Verification items for this drawing (mm, ordinates from the low corner). Round coordinates to 2 decimals unless told otherwise and drop trailing zeros. Write each loop counter-clockwise with the first axis right and the second up, starting at its lowest first coordinate (ties: lowest second). Pieces come first, ordered by that corner, then holes. Notation, with made-up numbers: (64, 7.5) -> (113, 7.5) arc R18 cw to (113, 33.5) -> close; hole circle Ø5 at (63.25, 17.25). An arc over 180 degrees is marked (long way). One line per item, written item: value.
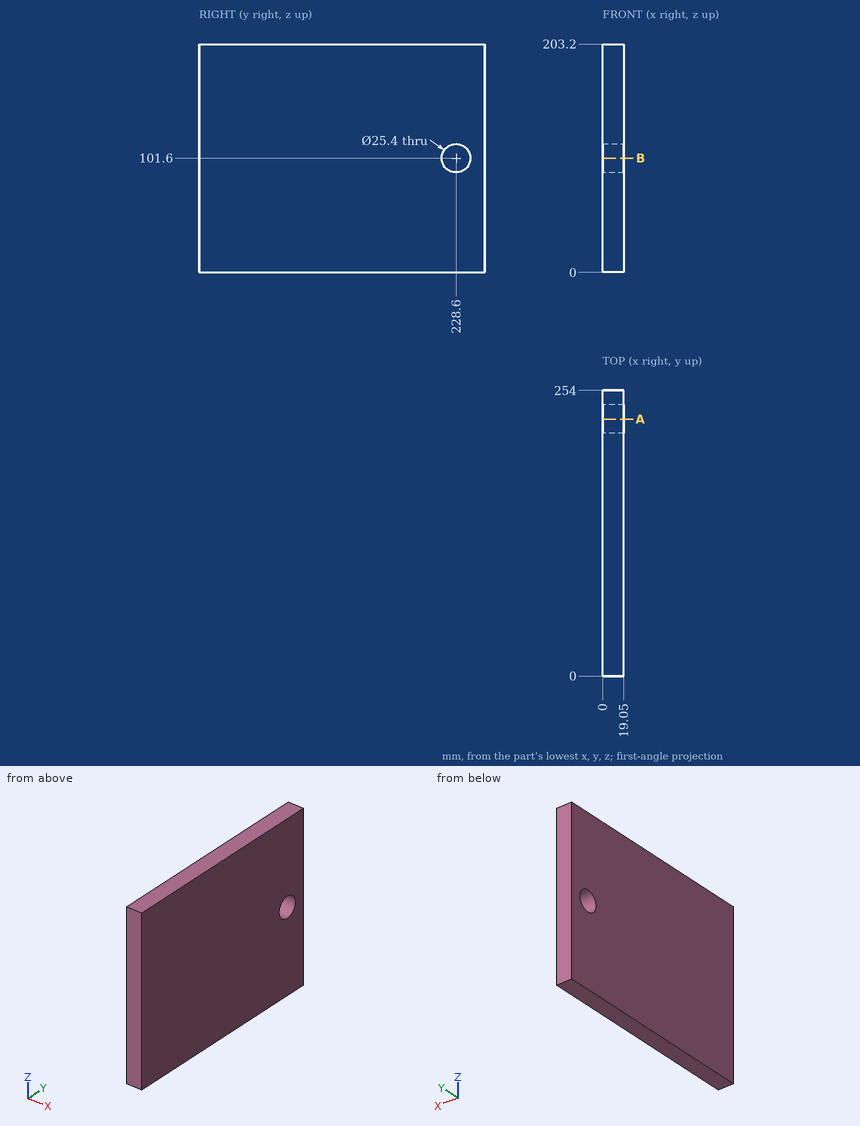
Item 1: Material ranges on line 1 along Y through (x, z) = (4.25, 101.6), recorded low to high.
Result set:
line 1: 0 to 215.9, 241.3 to 254
Item 2: Depth check by flat-ended pin: pin 1 (15 mm diameter, centred on y = 228.6, z = 101.6, fed in from -X). Enter the tip coordinate at first touch or a pass-through.
Result set:
pin 1: through
Item 3: Sectioned sample at A-A (y = 228.6). Enter the section's corners in (x, z), then the cut area to 3 significant figures.
Result set:
outline: (0, 0) -> (19.05, 0) -> (19.05, 88.9) -> (0, 88.9) -> close; (0, 114.3) -> (19.05, 114.3) -> (19.05, 203.2) -> (0, 203.2) -> close
area: 3,390 mm^2
Item 4: Sectioned sample at B-B (z = 101.6). Enter the section's corners in (x, y), then the cut area to 3 significant figures.
Result set:
outline: (0, 0) -> (19.05, 0) -> (19.05, 215.9) -> (0, 215.9) -> close; (0, 241.3) -> (19.05, 241.3) -> (19.05, 254) -> (0, 254) -> close
area: 4,350 mm^2
